Input: part model. Units: mm. Frame: model coordinates. Face numbers are marked on the shaded views. A direction names the side the tool comes from. Coordinates: 2 decimals unless noted, no trailing zeros. Write each loop counter-clockwise with the first axis right and the second up, starting at its lowest first coordinate (ties: lowest second). Pieces come first, ordered by that corner, then holes.
1) Line query: L1, parallel to X at y = 53, z = 26; L2, parallel to Y at x = -26.5, z = 29; L3, parallel to Z at x = -24.5, y = 41. Output: solid intervals per line, ascending.
2) Section query A-A (z = 37.5). Output: boundary loops of the cut face in (x, y).
3) Section query D-D (z = -37). Output: boundary loops of the cut face in (x, y).
4) Section query B-B (x = -40). Output: boundary loops of the cut face in (y, z), then the cut area to 3 significant figures.
5) Section query C-C (y = 55.5). Output: boundary loops of the cut face in (x, z), then the cut area to 3 significant figures.
6) Set-up query: the marked faces 1, 2 and 3. Return all of +Z, -Z, +X, -X, +Y, -Y with unobstructed straight access to the full face (end or side cutting, diameter ignored); none if empty.
7) Pin query (flat end, axial travel): pin 1 Ø9 at (x, z) = (36, 38.5) entering from +Y; pin 2 Ø1 at (x, y) = (40, 64.5) entering from +Z; pin 3 Ø9 at (y, z) = (62, 43) entering from +X. Return the tip coordinate at first contact, or that it passes through.
from build123d import *

# Parameters (mm, degrees)
SKETCH3_W               = 100
SKETCH3_H               = 150
BOSS_EXTRUDE2_DEPTH     = 80
CUT_EXTRUDE4_DEPTH      = 100
CUT_EXTRUDE5_DEPTH      = 149.408220797
CUT_EXTRUDE5_DEPTH_BACK = 30
SKETCH4_5_W             = 51.304080983
SKETCH4_5_H             = 30
SKETCH6_W               = 40
SKETCH6_H               = 50
CUT_EXTRUDE6_DEPTH      = 30


with BuildPart() as part:
    # Sketch3 → Boss-Extrude2 (new body)
    with BuildSketch(Plane(origin=(0, 0, 0), x_dir=(1, 0, 0), z_dir=(0, 1, 0))):
        Rectangle(SKETCH3_W, SKETCH3_H)
    extrude(amount=BOSS_EXTRUDE2_DEPTH)

    # Sketch4 → Cut-Extrude4 (cut)
    with BuildSketch(Plane(origin=(50, 0, 0), x_dir=(0, 0, -1), z_dir=(1, 0, 0))):
        Polygon((75, 80), (6.304080983, 80), (75, 40), align=None)
    extrude(amount=-CUT_EXTRUDE4_DEPTH, mode=Mode.SUBTRACT)

    # Sketch4<5> → Cut-Extrude5 (cut, two sides: drawn at the far end of the back side and taken through both)
    with BuildSketch(Plane(origin=(50, 0, 0), x_dir=(0, 0, -1), z_dir=(1, 0, 0)).offset(-CUT_EXTRUDE5_DEPTH_BACK)):
        with Locations((-49.347959508, 65)):
            Rectangle(SKETCH4_5_W, SKETCH4_5_H)
    extrude(amount=CUT_EXTRUDE5_DEPTH + CUT_EXTRUDE5_DEPTH_BACK, mode=Mode.SUBTRACT)

    # Sketch6 → Cut-Extrude6 (cut)
    with BuildSketch(Plane(origin=(0, 80, 0), x_dir=(1, 0, 0), z_dir=(0, 1, 0))):
        with Locations((-30, -50)):
            Rectangle(SKETCH6_W, SKETCH6_H)
    extrude(amount=-CUT_EXTRUDE6_DEPTH, mode=Mode.SUBTRACT)


solid = part.part
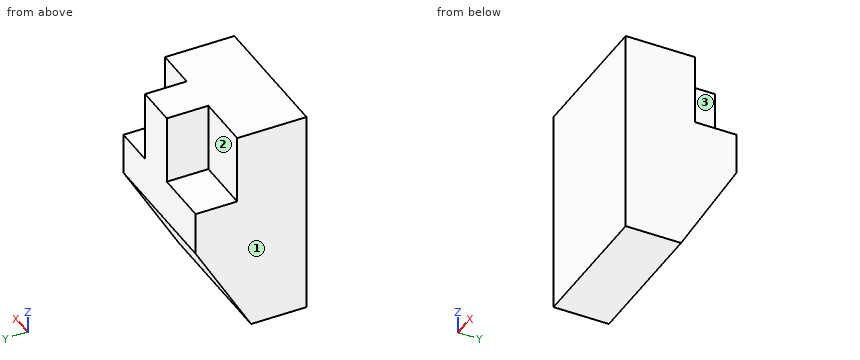
Answer:
1. L1: x = -10 to 20
1. L2: y = 0 to 50
1. L3: z = -73.28 to 75
2. outline: (-50, 0) - (50, 0) - (50, 50) - (20, 50) - (20, 80) - (-10, 80) - (-10, 50) - (-50, 50) - close
3. outline: (-50, 0) - (50, 0) - (50, 62.13) - (-50, 62.13) - close
4. outline: (0, -75) - (40, -75) - (80, -6.3) - (80, 25) - (50, 25) - (50, 75) - (0, 75) - close
4. area: 9,130 mm2
5. outline: (-50, -48.38) - (50, -48.38) - (50, 23.7) - (20, 23.7) - (20, 75) - (-10, 75) - (-10, 25) - (-50, 25) - close
5. area: 8,800 mm2
6. face 1: +Z, -Z, -X, +Y, -Y
6. face 2: +Z, -X, +Y
6. face 3: +Z, +X, +Y
7. pin 1: stops at y = 50
7. pin 2: stops at z = 23.7
7. pin 3: stops at x = 20
